Design review of the part built by this model. Coordinates are the model's own, in mm. Face numbers are marked on the shaded views. A direction names the side the tool comes from. Give positions to 0.01 mm unless a question says otherwise; leave off trailing zeros. Order: outer loops, then holes, each group sorted by start corner. A loop starts at its lowest first (then second) coordinate and runs counter-clockwise, first axis right, second up.
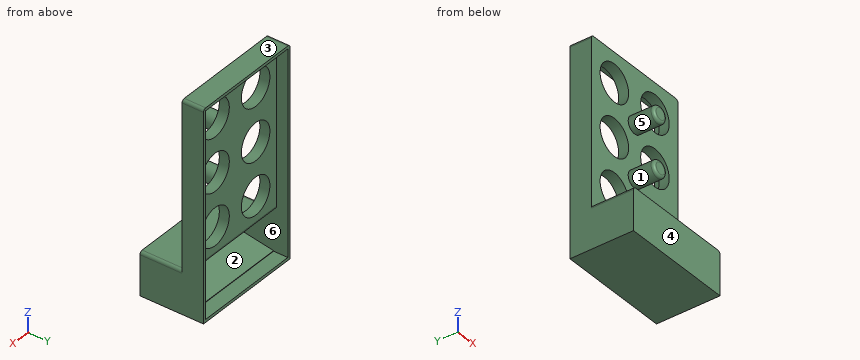
Autodesk Inventor part; units mm, degrees
ref_plane "YZ Plane" through (0, 0, 0) normal (1, 0, 0) x (0, 1, 0)
ref_plane "XY Plane" through (0, 0, 0) normal (0, 0, 1) x (1, 0, 0)
sketch "Sketch1" plane through (0, 0, 0) normal (0, 1, 0) x (-1, 0, 0)
  line L0 (25.9, 0) -> (-25.9, 0)
  line L1 (0, -25.9) -> (0, 25.9)
  circle A0 centre (0, 0) radius 18.5 construction
  circle A1 centre (0, 0) radius 13 construction
  dimension "d0" = 37
  dimension "d1" = 26
sketch "Sketch2" plane through (0, 0, 0) normal (0, 1, 0) x (-1, 0, 0)
  line L0 (36.8, 0) -> (-73.8, 0)
  line L1 (0, -44.2) -> (0, 118.2)
  line L2 (-58, 95) -> (-58, -21)
  line L3 (-58, -21) -> (21, -21)
  line L4 (21, -21) -> (21, 95)
  line L5 (-58, 95) -> (21, 95)
  circle A0 centre (-37, 0) radius 18.5 construction
  circle A1 centre (-37, 37) radius 18.5 construction
  circle A2 centre (-37, 74) radius 18.5 construction
  point P0 (0, 0)
  dimension "d29" = 21
  dimension "d30" = 95
  dimension "d109" = 58
  dimension "d110" = 21
  dimension "d111" = 37
  dimension "d112" = 37
  dimension "d113" = 37
  dimension "d114" = 37
  dimension "d115" = 37
  dimension "d116" = 37
  dimension "d117" = 37
  dimension "d118" = 37
extrude "Extrusion1" add sketch "Sketch2" along normal blind 7
sketch "Sketch6" plane through (0, 0, 0) normal (0, 1, 0) x (-1, 0, 0)
  line L0 (21, -21) -> (-58, -21)
  line L1 (21, 95) -> (21, -21)
  line L2 (-58, -21) -> (21, -21)
  line L3 (21, -21) -> (21, 95)
  line L4 (-58, 95) -> (-58, -21)
  line L5 (80.1765, 0) -> (-86.8627, 0)
  line L6 (0, -44.2) -> (0, 118.2)
  line L7 (21, 95) -> (-58, 95)
  line L8 (-53, 95) -> (-53, 0)
  line L9 (53, 0) -> (53, 95)
  line L10 (53, 95) -> (21, 95)
  line L11 (-58, 95) -> (-58, -21)
  line L12 (-58, 95) -> (-53, 95)
  arc A0 (37, -16) -> (53, 0) centre (37, 0) ccw
  arc A1 (-53, 0) -> (-37, -16) centre (-37, 0) ccw
  line L13 (37, -16) -> (-39.8141, -16)
  point P0 (0, 0)
  point P1 (-16, 0)
  dimension "d101" = 53
  dimension "d102" = 53
  dimension "d103" = 32
  dimension "d104" = 32
extrude "Extrusion5" [suppressed]
sketch "Sketch4" plane through (0, 0, 0) normal (0, 0, 1) x (1, 0, 0)
  line L0 (-55.5, 0) -> (55.5, 0)
  line L1 (55.5, 0) -> (55.5, -2.5)
  line L2 (55.5, -2.5) -> (-55.5, -2.5)
  line L3 (-55.5, -2.5) -> (-55.5, 0)
  line L4 (-77.7, 0) -> (77.7, 0)
  line L5 (0, -3) -> (0, 0.5)
  point P0 (0, 0)
  dimension "d10" = 111
  dimension "d11" = 2.5
extrude "Extrusion6" [suppressed]
sketch "Sketch5" plane through (0, 0, 0) normal (0, 1, 0) x (-1, 0, 0)
  circle A0 centre (0, 0) radius 18.5 construction
  circle A1 centre (0, 0) radius 18.5 construction
  line L0 (77.7, 0) -> (-77.7, 0)
  line L1 (0, -28.9) -> (0, 26.4)
  line L2 (-55.5, -21) -> (55.5, -21)
  line L3 (55.5, -21) -> (55.5, -18.5)
  line L4 (55.5, -18.5) -> (-55.5, -18.5)
  line L5 (-55.5, -18.5) -> (-55.5, -21)
  dimension "d25" = 111
  dimension "d26" = 21
extrude "Extrusion7" [suppressed]
sketch "Sketch7" plane through (0, 0, 0) normal (0, 0, 1) x (1, 0, 0)
  line L0 (-55.5, 0) -> (55.5, 0)
  line L1 (55.5, 0) -> (55.5, -2.5)
  line L2 (55.5, -2.5) -> (-55.5, -2.5)
  line L3 (-55.5, -2.5) -> (-55.5, 0)
  line L4 (58, 0) -> (-21, 0)
  line L5 (-79.2, 0) -> (86.7, 0)
  line L6 (0, -3) -> (0, 0.5)
  point P0 (-16, 0)
  point P1 (16, 0)
  point P2 (53, 0)
  point P3 (-53, 0)
  dimension "d53" = 2.5
  dimension "d54" = 55.5
extrude "Extrusion8" [suppressed]
sketch "Sketch8" plane through (0, 0, 0) normal (0, 1, 0) x (-1, 0, 0)
  circle A0 centre (0, 0) radius 13
  dimension "d34" = 26
extrude "Extrusion9" cut sketch "Sketch8" along normal through all
pattern_linear "Rectangular Pattern1" count 3 spacing 37 along (0, 0, 1) count 2 spacing 37 along (1, 0, 0) of "Extrusion9"
sketch "Sketch9" plane through (0, 7, 0) normal (0, 1, 0) x (1, 0, 0)
  circle A0 centre (0, 0) radius 13
  circle A1 centre (0, 0) radius 15
  dimension "d40" = 26
  dimension "d41" = 30
extrude "Extrusion10" [suppressed]
sketch "Sketch10" plane through (0, 5, 0) normal (0, 1, 0) x (1, 0, 0)
  arc A0 (16, 0) -> (-16, 0) centre (0, 0) ccw
  line L0 (1.5, -18) -> (-1.5, -18)
  line L1 (-29.4, 0) -> (29.4, 0)
  line L2 (0, 36.3) -> (0, -70.8)
  line L3 (1.5, -12) -> (-1.5, -12)
  line L4 (1.5, -12) -> (1.5, -18)
  line L5 (-1.5, -18) -> (-1.5, -12)
  dimension "d48" = 3
  dimension "d49" = 12
  dimension "d50" = 6
extrude "Extrusion11" [suppressed]
ref_plane "Work Plane1" through (0, 5, 0) normal (0, 1, 0) x (-1, 0, 0)
sketch "Sketch12" plane through (0, 5, 0) normal (0, 1, 0) x (-1, 0, 0)
  line L0 (21, -21) -> (-58, -21)
  line L1 (-58, -21) -> (-58, -51)
  line L2 (-58, -51) -> (21, -51)
  line L3 (21, -51) -> (21, -21)
  line L4 (43.8, 0) -> (-80.8, 0)
  line L5 (0, -64.9) -> (0, 32.4)
  point P0 (0, 0)
  dimension "d62" = 30
  dimension "d123" = 58
  dimension "d124" = 21
  dimension "d125" = 21
extrude "Extrusion12" add sketch "Sketch12" against normal blind 34.5
sketch "Sketch13" plane through (0, 0, 0) normal (1, 0, 0) x (0, 1, 0)
  line L0 (-31.4, 0) -> (13.4, 0)
  line L1 (0, -62.5) -> (0, 32)
  line L2 (7, -19) -> (7, -49)
  line L3 (7, -49) -> (-25, -43.3575)
  line L4 (-25, -43.3575) -> (-25, -30.647)
  line L5 (7, -19) -> (-25, -30.647)
  point P0 (0, 0)
  dimension "d85" = 25
  dimension "d86" = 7
  dimension "d87" = 49
  dimension "d88" = 30
  dimension "d89" = 100
  dimension "d90" = 110
extrude "Extrusion14" cut sketch "Sketch13" against normal blind 19
sketch "Sketch14" plane through (0, 5, 0) normal (0, 1, 0) x (-1, 0, 0)
  line L0 (0, -80.2) -> (0, 124.2)
  line L1 (19, 93) -> (-56, 93)
  line L2 (-56, 93) -> (-56, -49)
  line L3 (-56, -49) -> (19, -49)
  line L4 (19, -49) -> (19, 93)
  line L5 (21, 95) -> (-58, 95)
  line L6 (-58, 95) -> (-58, -51)
  line L7 (-58, -51) -> (21, -51)
  line L8 (21, -51) -> (21, 95)
  line L9 (43.8, 0) -> (-80.8, 0)
  dimension "d91" = 51
  dimension "d92" = 95
  dimension "d95" = 93
  dimension "d96" = 49
  dimension "d119" = 58
  dimension "d120" = 21
  dimension "d121" = 56
  dimension "d122" = 19
extrude "Extrusion15" add sketch "Sketch14" along normal blind 10 contours L7 L6 L9 L2 L3 L0 | L0 L3 L4 L9 L8 L7 | L6 L5 L0 L1 L2 L9 | L9 L4 L1 L0 L5 L8
fillet "Fillet3" radius 2 2 edges at (58, 7.5, 95) (-21, 7.5, 95)
fillet "Fillet5" radius 2 2 edges at (58, -14.75, -21) (-21, -14.75, -21)
fillet "Fillet8" [suppressed]
extrude "Extrusion16" cut sketch "Sketch13" along normal blind 56
sketch "Sketch15" plane through (0, 0, 0) normal (0, 1, 0) x (-1, 0, 0)
  circle A0 centre (-18.5, 18.5) radius 5.875
  line L0 (27.075, 0) -> (-32.95, 0)
  line L1 (0, -34.475) -> (0, 77.35)
  circle A1 centre (-18.5, 55.5) radius 5.875
  point P0 (0, 0)
  dimension "d128" = 18.5
  dimension "d129" = 18.5
  dimension "d130" = 11.75
  dimension "d133" = 37
extrude "Extrusion17" add sketch "Sketch15" against normal blind 18
fillet "Fillet9" radius 2 2 edges at (24.375, -18, 55.5) (24.375, -18, 18.5)
fillet "Fillet10" radius 4 2 edges at (18.5, -25, -43.3575) (18.5, -25, -30.647)
fillet "Fillet11" radius 2 1 edges at (18.5, 7, -19)
sketch "Sketch16" plane through (-19, 0, 0) normal (1, 0, 0) x (0, 0, -1)
  circle A0 centre (34.9178, 2) radius 13
  line L0 (48.6473, 5) -> (43.9404, -21.6946)
  line L1 (-93, 15) -> (49, 15)
  line L2 (49.4247, 14.4011) -> (38.404, -16.7639)
  line L3 (38.404, -16.7639) -> (16.9247, 8.3628)
  line L4 (16.9247, 8.3628) -> (49.4247, 14.4011)
  line L5 (49, 5) -> (49, 15)
  line L6 (49, 11.3819) -> (46.2939, 13.8194)
  point P0 (0, 0)
  dimension "d163" = 26
  dimension "d164" = 32.5
equation "\"d115\" = d114"
equation "\"d117\" = d116"
equation "\"d118\" = d115"
equation "\"d102\" = d101"
properties part number "NespressoSpeedfiller-6X-long"
1. For pin 1 (3.5 mm diameter, centred on x = 1, z = -37.5, fed in from +Y); pin 2 (1.5 mm diameter, centred on x = 35, z = 16, fed in from +Y); pin 3 (15.5 mm diameter, centred on x = 0, z = 74, fed in from -Y); pin 4 (8.5 mm diameter, centred on x = 20, z = 18.5, fed in from -Y), all flat-tipped, find the tip position at first contact; note any pin that passes through.
Recorded:
pin 1: stops at y = -25
pin 2: stops at y = 7
pin 3: passes through
pin 4: stops at y = -18
2. Take a section at C-C (y = -6). State the section outline as (x, z) points (3 decimals), then the cut area to 3 significant figures.
Recorded:
outline: (-21, -51) - (58, -51) - (58, -23) arc R2 ccw to (56, -21) - (-19, -21) arc R2 ccw to (-21, -23) - close; circle Ø11.75 at (18.5, 18.5); circle Ø11.75 at (18.5, 55.5); hole (-19, -46.708) - (56, -46.708) - (56, -23.732) - (-19, -23.732) - close
area: 862 mm2
3. Take a section at A-A (x = 0). State how many separate pieces and enclosed holes the cut face has, then the cut area to 3 significant figures.
Recorded:
separate pieces: 4
enclosed holes: 0
area: 713 mm2
4. For line 1 along X through (y, z) = (5.75, 0); line 2 along X through (y, z) = (-4.5, -32); line 3 along Z through (x, y) = (37, 4.75), list the stretches that pass through material, from the lowest coordinate up.
Recorded:
line 1: x = -21 to -13, 13 to 24, 50 to 58
line 2: x = -21 to -19, 56 to 58
line 3: z = -51 to -48.6, -19.82 to -13, 13 to 24, 50 to 61, 87 to 95
5. Take a section at B-B (z = 74). State the section outline as (x, y) points.
Recorded:
outline: (-21, 0) - (-13, 0) - (-13, 7) - (-19, 7) - (-19, 15) - (-21, 15) - close; (13, 0) - (24, 0) - (24, 7) - (13, 7) - close; (50, 0) - (58, 0) - (58, 15) - (56, 15) - (56, 7) - (50, 7) - close
6. Machinability: for the marked faces 4, 5 and 6, which of the approach directions +Z, -Z, +X, -X, +Y, -Y give a long, thin tool a straight path to every point of the face, cutting with its end or side? Answer none if there is none.
Recorded:
face 4: +Z, -Z, +X, -X, -Y
face 5: -Y
face 6: +Y
7. Draft analysis for pull direction X (two halves, no side actions). For the marked faces 1, 2 and 3, state which applies: pulls with the +X half, pulls with the -X half, needs draft (parallel to the pull), parting line crosses it, or undercut.
Recorded:
face 1: parting line crosses it
face 2: undercut
face 3: needs draft
